The model under review builds one solid part; all positions refer to its coordinate system, in mm. A direction names the side the tool comes from. Give positions to 0.01 mm unless a question says otherwise; leave off trailing zeros. Order: outer loops, then holes, each group sorted by start corner. A loop starts at its lowest first (then second) coordinate and runs counter-clockwise, first axis right, second up.
```python
from build123d import *

# Parameters (mm, degrees)
F0_W     = 102
F0_H     = 25
F1_DEPTH = 7
F2_R     = 5
F3_T     = -2.5
F4_R     = 1
F5_R     = 3.75
F6_DEPTH = 3
F7_R     = 1.5
F8_DEPTH = 3


with BuildPart() as f1:
    # F0 (on Top) → F1 (new body)
    with BuildSketch(Plane.XY):
        Rectangle(F0_W, F0_H)
    extrude(amount=F1_DEPTH)

    # F2
    f2_edges = [f1.edges().sort_by_distance(p)[0] for p in [
        (-51, -12.5, 3.5),
        (-51, 12.5, 3.5),
        (51, -12.5, 3.5),
        (51, 12.5, 3.5),
    ]]
    fillet(f2_edges, radius=F2_R)

    # F3
    f3_openings = [f1.faces().sort_by_distance(p)[0] for p in [
        (0, 0, 7),
    ]]
    offset(amount=F3_T, openings=f3_openings)

    # F4
    f4_edges = [f1.edges().sort_by_distance(p)[0] for p in [
        (-48.5, 0, 2.5),
        (-47.767767, -9.267767, 2.5),
        (0, -10, 2.5),
        (47.767767, -9.267767, 2.5),
        (48.5, 0, 2.5),
        (47.767767, 9.267767, 2.5),
        (0, 10, 2.5),
        (-47.767767, 9.267767, 2.5),
        (0, 12.5, 7),
        (-49.535534, 11.035534, 7),
        (-51, 0, 7),
        (-49.535534, -11.035534, 7),
        (0, -12.5, 7),
        (49.535534, -11.035534, 7),
        (51, 0, 7),
        (49.535534, 11.035534, 7),
        (0, 10, 7),
        (47.767767, 9.267767, 7),
        (48.5, 0, 7),
        (47.767767, -9.267767, 7),
        (0, -10, 7),
        (-47.767767, -9.267767, 7),
        (-48.5, 0, 7),
        (-47.767767, 9.267767, 7),
        (0, 12.5, 0),
        (49.535534, 11.035534, 0),
        (-49.535534, 11.035534, 0),
        (51, 0, 0),
        (-51, 0, 0),
        (49.535534, -11.035534, 0),
        (-49.535534, -11.035534, 0),
        (0, -12.5, 0),
    ]]
    fillet(f4_edges, radius=F4_R)

    # F5 (on face) → F6 (join)
    with BuildSketch(Plane.XY.offset(2.5)):
        with Locations((-9.525, -6.985)):
            Circle(F5_R)
        with Locations((9.525, -6.985)):
            Circle(F5_R)
        with Locations((-28.575, 6.985)):
            Circle(F5_R)
        with Locations((28.575, 6.985)):
            Circle(F5_R)
    extrude(amount=F6_DEPTH)

    # F7 (on face) → F8 (cut, through all)
    with BuildSketch(Plane.XY.offset(5.5)):
        with Locations((-9.525, -6.985)):
            Circle(F7_R)
        with Locations((-28.575, 6.985)):
            Circle(F7_R)
        with Locations((9.525, -6.985)):
            Circle(F7_R)
        with Locations((28.575, 6.985)):
            Circle(F7_R)
    extrude(amount=-F8_DEPTH, mode=Mode.SUBTRACT)


solid = f1.part
```
1. Take a section at D-D (x = -29). Write out the cut boundary in (y, z).
2. Insertion check: pin 1 (7.5 mm diameter, centred on x = 8, y = -7, fed in from +Z); pin 2 (5.5 mm diameter, centred on x = -1, y = -3.5, fed in from +Z); pin 3 (2.5 mm diameter, centred on x = 9, y = -7, fed in from +Z). Each pin has a flat end and moves straight along its axis. Give the tip position at first contact, or say it passes through.
3. Take a section at C-C (x = 38.5). Write out the cut boundary in (y, z).
4. For faces 1 (the flat face through (-1, -10, 5)), 2 (the flat face through (-1, -12.5, 3)), list the 3-axis set-ups (+Z, -Z, +X, -X, +Y, -Y) from which the entire face can be reached by the end or side of a thin tool; tool diameter is ignored.
5. Take a section at A-A (y = 0.75). Write out the cut boundary in (x, z).
6. Take a section at B-B (z = 4.5). Write out the cut boundary in (x, y) (3 decimals), and give its area (3 significant figures).
7. Draft analysis for pull direction X (two halves, no side actions). For faces 3 (the flat face through (29, 7, 2.5)), 4 (the flat face through (51, 0, 3)), 5 (the flat face through (-1, 12.5, 3)), state which applies: pulls with the +X half, pulls with the -X half, needs draft (parallel to the pull), parting line crosses it, or undercut.
8. To check wall thickness, follow line 1 (Y direction, x = 5.5, z = 3.5); line 2 (X direction, y = 2, z = 4.5); line 3 (Y direction, x = 28, z = 5.25). State the ranges of each line that lie inside material, in increasing order.
Answer:
1. outline: (-12.5, 1) arc R1 ccw to (-11.5, 0) - (11.5, 0) arc R1 ccw to (12.5, 1) - (12.5, 6) arc R1 ccw to (11.5, 7) - (11, 7) arc R1 ccw to (10, 6) - (10, 5.5) - (8.42, 5.5) - (8.42, 2.5) - (5.55, 2.5) - (5.55, 5.5) - (3.26, 5.5) - (3.26, 2.5) - (-9, 2.5) arc R1 cw to (-10, 3.5) - (-10, 6) arc R1 ccw to (-11, 7) - (-11.5, 7) arc R1 ccw to (-12.5, 6) - close
2. pin 1: stops at z = 6.97
2. pin 2: stops at z = 2.5
2. pin 3: stops at z = 5.5
3. outline: (-12.5, 1) arc R1 ccw to (-11.5, 0) - (11.5, 0) arc R1 ccw to (12.5, 1) - (12.5, 6) arc R1 ccw to (11.5, 7) - (11, 7) arc R1 ccw to (10, 6) - (10, 3.5) arc R1 cw to (9, 2.5) - (-9, 2.5) arc R1 cw to (-10, 3.5) - (-10, 6) arc R1 ccw to (-11, 7) - (-11.5, 7) arc R1 ccw to (-12.5, 6) - close
4. face 1: +Z
4. face 2: +Z, -Z, +X, -X, -Y
5. outline: (-51, 1) arc R1 ccw to (-50, 0) - (50, 0) arc R1 ccw to (51, 1) - (51, 6) arc R1 ccw to (50, 7) - (49.5, 7) arc R1 ccw to (48.5, 6) - (48.5, 3.5) arc R1 cw to (47.5, 2.5) - (-47.5, 2.5) arc R1 cw to (-48.5, 3.5) - (-48.5, 6) arc R1 ccw to (-49.5, 7) - (-50, 7) arc R1 ccw to (-51, 6) - close
6. outline: (-51, -7.5) arc R5 ccw to (-46, -12.5) - (46, -12.5) arc R5 ccw to (51, -7.5) - (51, 7.5) arc R5 ccw to (46, 12.5) - (-46, 12.5) arc R5 ccw to (-51, 7.5) - close; hole (-48.5, -7.5) arc R2.5 ccw to (-46, -10) - (-11.755, -10) arc R3.75 cw (long way) to (-7.295, -10) - (7.295, -10) arc R3.75 cw (long way) to (11.755, -10) - (46, -10) arc R2.5 ccw to (48.5, -7.5) - (48.5, 7.5) arc R2.5 ccw to (46, 10) - (30.805, 10) arc R3.75 cw (long way) to (26.345, 10) - (-26.345, 10) arc R3.75 cw (long way) to (-30.805, 10) - (-46, 10) arc R2.5 ccw to (-48.5, 7.5) - close; hole circle Ø3 at (-28.575, 6.985); hole circle Ø3 at (-9.525, -6.985); hole circle Ø3 at (9.525, -6.985); hole circle Ø3 at (28.575, 6.985)
6. area: 733 mm2
7. face 3: undercut
7. face 4: pulls with the +X half
7. face 5: needs draft
8. line 1: y = -12.5 to -10, 10 to 12.5
8. line 2: x = -51 to -48.5, 48.5 to 51
8. line 3: y = -12.5 to -10, 3.28 to 5.6, 8.37 to 12.5
